Here's the drawing with two shaded views (mm, measured from the low corner). I have some questions. A direction names the side the tool comes from. Give positions to 0.01 mm unless a question says otherwise; leave off trailing zeros. Loops run counter-clockwise (first coordinate to the right, second up) from the corner with the lowest first, then second, coordinate; pieces in that order, holes last. Notation, with made-up numbers: (48, 17.5) - (106, 17.5) arc R5 ccw to (106, 22.5) - close; hole circle Ø9 at (-14, 76). An arc over 180 degrees is marked (long way). Answer as a JSON object with one key per item and string values. Group by question number.
Item 1: Which directions (+Z, -Z, +X, -X, +Y, -Y) give clear straight access to the entire face, cutting with the end or side of a thin tool? Please do the marked faces 1 and 2.
Item 2: Will this pin go through, and if not, where does the flat tip stop? pin 1 (5 mm diameter, centred on x = 22, y = 26, fed in from +Z).
Item 3: Please list where these lines run through material, in increasing order: L1, parallel to Y at x = 0.4, z = 44.45; L2, parallel to Y at x = 24.8, z = 10.16; L3, parallel to X at y = 25, z = 13.5.
Item 4: Suppose I cut it at A-A on y = 40.64. Write out the boundary of the cut face in (x, z).
Item 5: Suppose I cut it at D-D on z = 10.16. Write out the boundary of the cut face in (x, y).
Item 6: Suppose I cut it at C-C on x = 18.5. Write out the boundary of the cut face in (y, z), and give its area (3 significant figures).
Item 7: Suppose I cut it at B-B on z = 44.45. Count the separate pieces of the cut face and the enclosed holes in it, and give its area (3 significant figures).
Item 8: Thinking about a two-plate mould opening in Y: for the marked faces 3, 4 and 5, which applies, pulls with the +Y half, pulls with the -Y half, needs draft (parallel to the pull), parting line crosses it, or undercut?
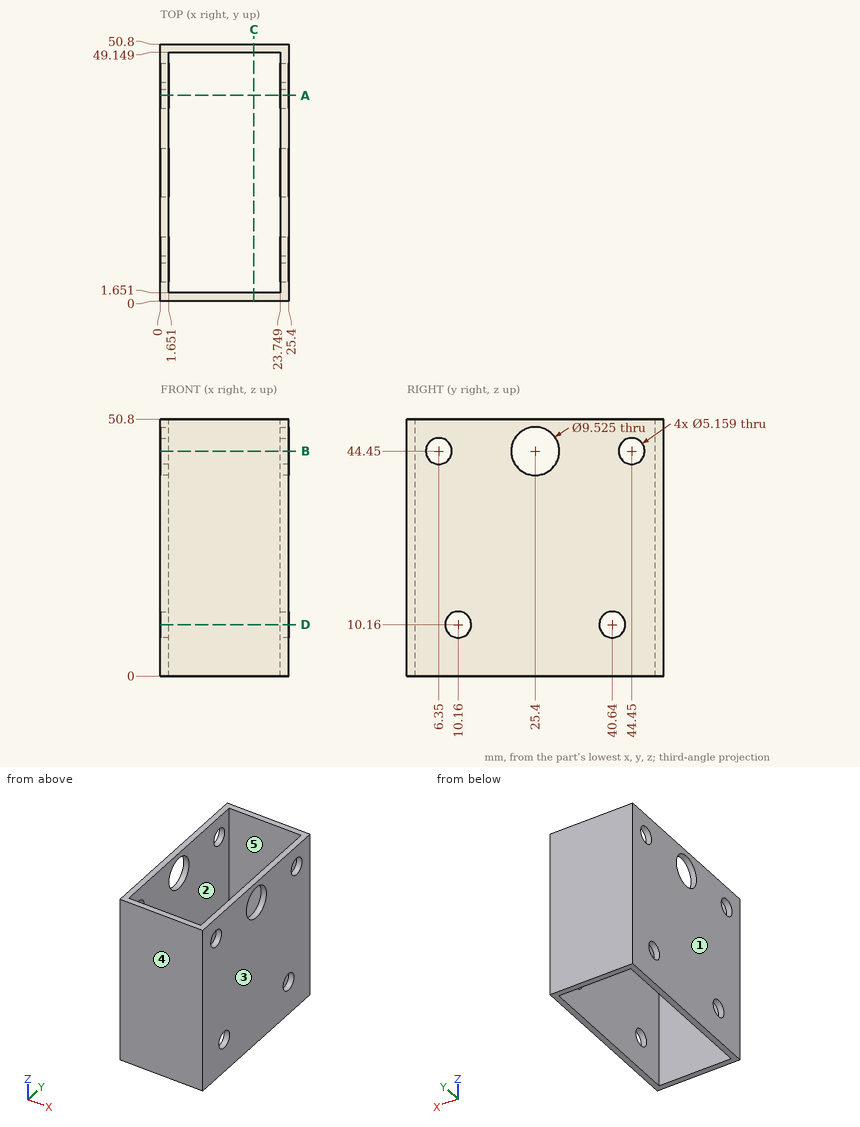
Worked out:
{
 "1": {"face 1": "+Z, -Z, -X, +Y, -Y", "face 2": "+Z, -Z"},
 "2": {"pin 1": "stops at z = 50.8"},
 "3": {"L1": "y = 0 to 3.77, 8.93 to 20.64, 30.16 to 41.87, 47.03 to 50.8", "L2": "y = 0 to 7.58, 12.74 to 38.06, 43.22 to 50.8", "L3": "x = 0 to 1.65, 23.75 to 25.4"},
 "4": {"outline": "(0, 0) - (1.65, 0) - (1.65, 7.58) - (0, 7.58) - close; (0, 12.74) - (1.65, 12.74) - (1.65, 50.8) - (0, 50.8) - close; (23.75, 0) - (25.4, 0) - (25.4, 7.58) - (23.75, 7.58) - close; (23.75, 12.74) - (25.4, 12.74) - (25.4, 50.8) - (23.75, 50.8) - close"},
 "5": {"outline": "(0, 0) - (25.4, 0) - (25.4, 7.58) - (23.75, 7.58) - (23.75, 1.65) - (1.65, 1.65) - (1.65, 7.58) - (0, 7.58) - close; (0, 12.74) - (1.65, 12.74) - (1.65, 38.06) - (0, 38.06) - close; (0, 43.22) - (1.65, 43.22) - (1.65, 49.15) - (23.75, 49.15) - (23.75, 43.22) - (25.4, 43.22) - (25.4, 50.8) - (0, 50.8) - close; (23.75, 12.74) - (25.4, 12.74) - (25.4, 38.06) - (23.75, 38.06) - close"},
 "6": {"outline": "(0, 0) - (1.65, 0) - (1.65, 50.8) - (0, 50.8) - close; (49.15, 0) - (50.8, 0) - (50.8, 50.8) - (49.15, 50.8) - close", "area": "168 mm2"},
 "7": {"separate pieces": "6", "enclosed holes": "0", "area": "175 mm2"},
 "8": {"face 3": "needs draft", "face 4": "pulls with the -Y half", "face 5": "undercut"}
}
